from build123d import *

# Parameters (mm, degrees)
F0_W     = 406.4
F0_H     = 101.6
F1_DEPTH = 12.7
F2_W     = 406.4
F2_H     = 7.874
F3_DEPTH = 9.652
F5_D     = 8.001
F5_DEPTH = 9.652
F5_TIP   = 2.4037429064


with BuildPart() as f1:
    # F0 (on Right) → F1 (new body)
    with BuildSketch(Plane.YZ):
        Rectangle(F0_W, F0_H)
    extrude(amount=F1_DEPTH)

    # F2 (on face) → F3 (cut)
    with BuildSketch(Plane.YZ.offset(12.7)):
        with Locations((0, -40.513)):
            Rectangle(F2_W, F2_H)
    extrude(amount=-F3_DEPTH, mode=Mode.SUBTRACT)

    # F5
    with Locations(Plane.YZ.offset(12.7)):
        with Locations((-196.85, 25.4), (-196.85, -12.7), (196.85, 25.4), (196.85, -12.7)):
            Hole(F5_D / 2, depth=F5_DEPTH)
            with Locations((0, 0, -(F5_DEPTH + F5_TIP / 2))):  # 118° drill point
                Cone(0, F5_D / 2, F5_TIP, mode=Mode.SUBTRACT)


solid = f1.part
Could you check a few things on this model? Use its own coordinates, in mm. A direction names the side the tool comes from. Give positions to 0.01 mm unless a question says otherwise; leave off trailing zeros. Write each loop counter-clockwise with the first axis right and the second up, starting at its lowest first coordinate (ties: lowest second). Pieces come first, ordered by that corner, then holes. Notation, with made-up numbers: (83, 51.5) -> (118, 51.5) arc R12 ccw to (118, 63.5) -> close; hole circle Ø2 at (32, -32). An arc over 180 degrees is marked (long way). Write each question's results on one line, items separated by ' | '. Start each with the question number.
Q1. I need wall thicknesses on probe 1 along Y at (x, z) = (9.5, -12.7); probe 2 along Z at (x, y) = (7.5, -196.85); probe 3 along Z at (x, y) = (9.5, -1). Which ranges of each line are inside material? Lowest first, please.
Q2. I'm going to push flat-ended pins straight in: pin 1 Ø6.5 at (y, z) = (-196.85, 25.4) entering from +X; pin 2 Ø5 at (y, z) = (196.85, -12.7) entering from +X. Where does each tip first touch, or does it pass through?
Q3. We'd pull the mould along Z, two halves only. Please class faces 4 (the face through (6, -203.2, -1)), 5 (the face through (6, -3, -50.8)), 6 (the face through (7.806, -195.983, 21.495)): +Z half, -Z half, draft (parallel to the pull), parting line (faces both ways), or undercut.
Q4. Suppose I cut it at B-B, the plane y = 173. List the corners of the cut face in (x, z) for me, and give its area (3 significant figures).
Q5. Suppose I cut it at C-C, the plane z = -40.5. List the corners of the cut face in (x, y) for me.
Q6. Suppose I cut it at A-A, the plane x = 9.25. List the corners of the cut face in (y, z) for me.
Q7. Which directions (+Z, -Z, +X, -X, +Y, -Y) give clear straight access to the entire face, cutting with the end or side of a thin tool? Please do faces 1 (the face through (3.048, -3, -40)), 2 (the face through (0, -3, 1)), 3 (the face through (7.806, 200.847, 25.576)).
Outcome:
1) probe 1: -203.2 to -200.85, -192.85 to 192.85, 200.85 to 203.2 | probe 2: -50.8 to -44.45, -36.58 to -16.7, -8.7 to 21.4, 29.4 to 50.8 | probe 3: -50.8 to -44.45, -36.58 to 50.8
2) pin 1: x = 2.6 | pin 2: x = 2.15
3) face 4: draft | face 5: -Z half | face 6: undercut
4) outline: (0, -50.8) -> (12.7, -50.8) -> (12.7, -44.45) -> (3.05, -44.45) -> (3.05, -36.58) -> (12.7, -36.58) -> (12.7, 50.8) -> (0, 50.8) -> close | area: 1,210 mm2
5) outline: (0, -203.2) -> (3.05, -203.2) -> (3.05, 203.2) -> (0, 203.2) -> close
6) outline: (-203.2, -50.8) -> (203.2, -50.8) -> (203.2, -44.45) -> (-203.2, -44.45) -> close; (-203.2, -36.58) -> (203.2, -36.58) -> (203.2, 50.8) -> (-203.2, 50.8) -> close; hole circle Ø8 at (-196.85, -12.7); hole circle Ø8 at (-196.85, 25.4); hole circle Ø8 at (196.85, -12.7); hole circle Ø8 at (196.85, 25.4)
7) face 1: +X, +Y, -Y | face 2: +Z, -Z, -X, +Y, -Y | face 3: +X
